Here's how the part is built. I have some questions about the finished solid (model axes, mm). A direction names the side the tool comes from. Coordinates: 2 decimals unless noted, no trailing zeros. Write each loop counter-clockwise with the first axis right and the second up, starting at its lowest first coordinate (ties: lowest second). Pieces come first, ordered by that corner, then holes. Notation, with made-up numbers: (36, -35) -> (66, -35) arc R20 ccw to (66, -19) -> close; hole circle Ø3 at (1, 14.5). An arc over 180 degrees is marked (long way). Put each result on its own line as item: value. Start each with the question number.
Item 1: On a 3-axis mill with a long thin cutter (end or side, diameter ignored), from which of +Z, -Z, +X, -X, +Y, -Y can I reach the whole of each face in a straight line? I mean faces 1 (the face through (15, 0, 18)), 2 (the face through (-1, -5, 2)), 3 (the face through (25, 2, 2)), 4 (the face through (0, 4, 20)), 5 (the face through (-15, 0, 18)). Say none if no direction works.
Item 2: I want a section at B-B, the plane x = 0. List the corners of the cut face in (y, z) for me, then the cut area to 3 significant figures.
Item 3: I want a section at D-D, the plane z = 27. List the corners of the cut face in (x, y) for me, then the cut area to 3 significant figures.
Item 4: For pin 1 (8.5 mm diameter, centred on x = 3, z = 26, fed in from -Y); pin 2 (3 mm diameter, centred on y = 2, z = 9.5, fed in from -X); pin 3 (3 mm diameter, centred on y = 2, z = 21, fed in from +X), each with a flat end and sliding along its axis, tell me the tip position at first contact or that it passes through.
Item 5: I want a section at A-A, the plane y = 0.25. List the corners of the cut face in (x, z) for me.
Item 6: I want a section at C-C, the plane y = -3. List the corners of the cut face in (x, z) for me.
Item 7: I need wall thicknesses on line 1 (Z direction, x = 0, y = 0.5); line 2 (X direction, y = -2, z = 4.5); line 3 (Z direction, x = -28, y = 4). Which ranges of each line are inside material? Lowest first, please. Write a range as [from, to].
Item 8: If we mould it in two halves opening along Z, with no side actions, what happens to faces 6 (the face through (-14.14, 0.06, 33.1)), 7 (the face through (-0.351, 0.056, 29.677)), 8 (the face through (-18.22, -0.06, 1.97))? For each: released by +Z, released by -Z, zero draft, split by the parting line, or undercut.
from build123d import *

# Parameters (mm, degrees)
F0_W        = 80
F0_H        = 10
F2_DEPTH    = 4
F1_W        = 30
F1_H        = 34
F1_R        = 2.7
F3_DEPTH    = 4
F4_T1_DEPTH = 30
F4_T3_DEPTH = 30
F4_T5_DEPTH = 23
F4_T7_DEPTH = 23


# Not quite as in the source:
# - a fillet or chamfer that OpenCascade refuses, or shapes differently, is made with other operations: its cross-section is extruded or revolved along the edge and cut away or added


with BuildPart() as f2:
    # F0 (on Top) → F2 (new body)
    with BuildSketch(Plane.XY):
        Rectangle(F0_W, F0_H)
        with BuildLine():
            ThreePointArc((-29.8963663541, -2.000000095), (-31.8970374873, -0.0504918144), (-30, 1.999999905))
            Line((-30, 1.999999905), (-20, 1.999999905))
            ThreePointArc((-20, 1.999999905), (-18.2234549617, -0.1070915702), (-20.226663407, -2.000000095))
            Line((-20.226663407, -2.000000095), (-29.8963663541, -2.000000095))
        make_face(mode=Mode.SUBTRACT)
        with BuildLine():
            ThreePointArc((20.0609671511, -2.000000095), (18.0607348524, -0.030022587), (20, 1.999999905))
            Line((20, 1.999999905), (30, 1.999999905))
            ThreePointArc((30, 1.999999905), (31.7352004336, -0.1259018267), (29.7306719608, -2.000000095))
            Line((29.7306719608, -2.000000095), (20.0609671511, -2.000000095))
        make_face(mode=Mode.SUBTRACT)
    extrude(amount=F2_DEPTH)

    # F1 (on Front) → F3 (join, symmetric)
    with BuildSketch(Plane.XZ):
        with Locations((0, 17)):
            Rectangle(F1_W, F1_H)
        with Locations((0, 27)):
            Circle(F1_R, mode=Mode.SUBTRACT)
    extrude(amount=F3_DEPTH, both=True)

    # F4: fillet of radius 3 on 4 edges, made by hand

    # F4_s2 → F4_t1 (join)
    with BuildSketch(Plane.YZ.offset(-15)):
        with BuildLine():
            ThreePointArc((5, 4), (4.2613872125, 5.0113231061), (4, 6.2360679775))
            Line((4, 6.2360679775), (4, 4))
            Line((4, 4), (5, 4))
        make_face()
    extrude(amount=F4_T1_DEPTH)

    # F4_s4 → F4_t3 (join)
    with BuildSketch(Plane.YZ.offset(-15)):
        with BuildLine():
            ThreePointArc((-4, 6.2360679775), (-4.2613872125, 5.0113231061), (-5, 4))
            Line((-5, 4), (-4, 4))
            Line((-4, 4), (-4, 6.2360679775))
        make_face()
    extrude(amount=F4_T3_DEPTH)

    # F4_s6 → F4_t5 (cut)
    with BuildSketch(Plane.XZ.offset(-11.5)):
        with BuildLine():
            ThreePointArc((15, 31), (14.1213203436, 33.1213203436), (12, 34))
            Line((12, 34), (15, 34))
            Line((15, 34), (15, 31))
        make_face()
    extrude(amount=F4_T5_DEPTH, mode=Mode.SUBTRACT)

    # F4_s8 → F4_t7 (cut)
    with BuildSketch(Plane.XZ.offset(-11.5)):
        with BuildLine():
            ThreePointArc((-15, 31), (-14.1213203436, 33.1213203436), (-12, 34))
            Line((-12, 34), (-15, 34))
            Line((-15, 34), (-15, 31))
        make_face()
    extrude(amount=F4_T7_DEPTH, mode=Mode.SUBTRACT)


solid = f2.part
Calculated:
1. face 1: +Z, +X, +Y, -Y
1. face 2: +Z, -Z, +X, -X, -Y
1. face 3: +Z, -Z
1. face 4: +Z, +X, -X, +Y
1. face 5: +Z, -X, +Y, -Y
2. outline: (-5, 0) -> (5, 0) -> (5, 4) arc R3 cw to (4, 6.24) -> (4, 24.3) -> (-4, 24.3) -> (-4, 6.24) arc R3 cw to (-5, 4) -> close; (-4, 29.7) -> (4, 29.7) -> (4, 34) -> (-4, 34) -> close
2. area: 238 mm2
3. outline: (-15, -4) -> (-2.7, -4) -> (-2.7, 4) -> (-15, 4) -> close; (2.7, -4) -> (15, -4) -> (15, 4) -> (2.7, 4) -> close
3. area: 197 mm2
4. pin 1: stops at y = -4
4. pin 2: stops at x = -15
4. pin 3: stops at x = 15
5. outline: (-40, 0) -> (-31.88, 0) -> (-31.88, 4) -> (-40, 4) -> close; (-18.24, 0) -> (18.08, 0) -> (18.08, 4) -> (15, 4) -> (15, 31) arc R3 ccw to (12, 34) -> (-12, 34) arc R3 ccw to (-15, 31) -> (-15, 4) -> (-18.24, 4) -> close; (31.73, 0) -> (40, 0) -> (40, 4) -> (31.73, 4) -> close; hole circle Ø5.4 at (0, 27)
6. outline: (-40, 0) -> (40, 0) -> (40, 4) -> (15, 4) -> (15, 31) arc R3 ccw to (12, 34) -> (-12, 34) arc R3 ccw to (-15, 31) -> (-15, 4) -> (-40, 4) -> close; hole circle Ø5.4 at (0, 27)
7. line 1: z = [0, 24.3], [29.7, 34]
7. line 2: x = [-15, 15]
7. line 3: z = [0, 4]
8. face 6: released by +Z
8. face 7: undercut
8. face 8: zero draft
